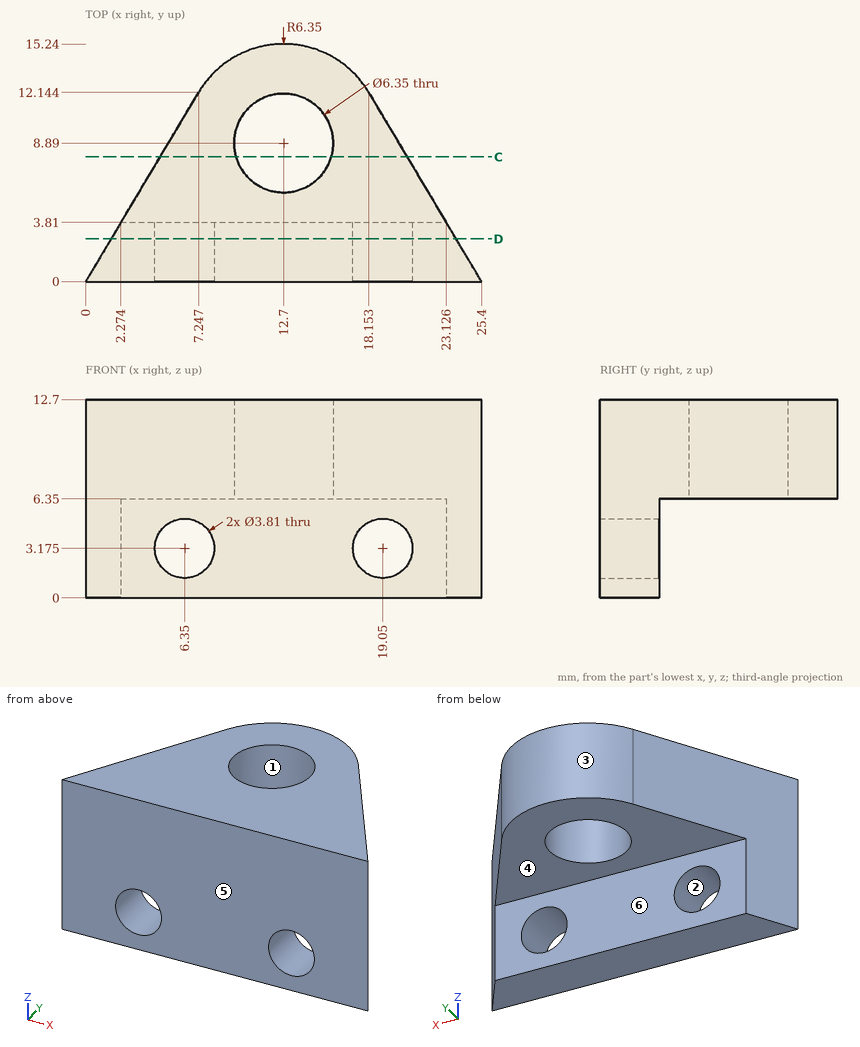
Geometry check sheet. Reference: drawing and pictorial views, mm from the part's lowest x, y, z. A direction names the side the tool comes from. Coordinates: 2 decimals unless noted, no trailing zeros. Order: outer loops, then holes, each group sorted by start corner. A loop starts at its lowest first (then second) coordinate and runs counter-clockwise, first axis right, second up. Notation, with made-up numbers: (-21, -15) -> (23, -15) arc R26 cw to (23, 17) -> close; hole circle Ø9 at (19, 73). An arc over 180 degrees is marked (long way). Use CSV: the item, a comma, the result in double quotes. Start each with the question number.
Q1. Draft check along X on the marked faces 1, 2, 3 and 4. Enter one of: +X half, -X half, draft (parallel to the pull), parting line (faces both ways), or undercut.
Q2. Thickness scan on line 1 along X through (y, z) = (3.5, 1.5) (1 decimal); line 2 along Z through (x, y) = (6.35, 2.8); line 3 along Z through (x, y) = (8.25, 10.5). Record the ranges inside material, lowest first.
Q3. Section check D-D, the plane y = 2.75. Give the number of separate pieces and of enclosed holes in the cut face, and give its area (3 significant figures).
Q4. Section check C-C, the plane y = 8. Record the cut outline in (x, z).
Q5. Depth check by flat-ended pin: P1, Ø1, axis at x = 11.5, z = 11.5, coming from the -Y side; P2, Ø2, axis at y = 4, z = 4, coming from the +X side; P3, Ø1.5, axis at y = 13, z = 11, coming from the +X side; P4, Ø4, axis at x = 22.5, z = 6, coming from the +Y side. Enter the tip coordinate at first touch or a pass-through.
Q6. Tool access check on the marked faces 5 and 6. Record the directions out of +Z, -Z, +X, -X, +Y, -Y that give a thin tool (end or side, any length) a straight path to the whole face; none if there is none.
Returned:
1,face 1,"undercut"
1,face 2,"undercut"
1,face 3,"parting line"
1,face 4,"draft"
2,line 1,"x = 2.1 to 5.4, 7.3 to 18.1, 20 to 23.3"
2,line 2,"z = 0 to 1.27, 5.08 to 12.7"
2,line 3,"z = 6.35 to 12.7"
3,separate pieces,"1"
3,enclosed holes,"2"
3,area,"258 mm^2"
4,outline,"(4.77, 6.35) -> (9.65, 6.35) -> (9.65, 12.7) -> (4.77, 12.7) -> close; (15.75, 6.35) -> (20.63, 6.35) -> (20.63, 12.7) -> (15.75, 12.7) -> close"
5,P1,"stops at y = 0"
5,P2,"stops at x = 23.61"
5,P3,"stops at x = 18.09"
5,P4,"stops at y = 8.16"
6,face 5,"+Z, -Z, +X, -X, -Y"
6,face 6,"-Z, +X, -X, +Y"
